from build123d import *

# Parameters (mm, degrees)
BOSS_EXTRUDE2_DEPTH     = 20
CUT_EXTRUDE1_DEPTH      = 4.016802691
CUT_EXTRUDE1_DEPTH_BACK = 7.783143762
FILLET1_R               = 3


with BuildPart() as part:
    # Sketch2 → Boss-Extrude2 (new body)
    with BuildSketch(Plane(origin=(0, 0, 0), x_dir=(1, 0, 0), z_dir=(0, 1, 0))):
        Polygon((0, 0), (-64, 6.783143762), (-64, 3.766341072), (0, -3.016802691), (64.316188922, 3.799852867), (64, 6.783143762), align=None)
    extrude(amount=BOSS_EXTRUDE2_DEPTH)

    # Sketch3 → Cut-Extrude1 (cut, two sides)
    with BuildSketch(Plane.XY) as cut_extrude1_sk:
        Polygon((0, 7.890942367), (-64, 5.798881402), (-64, 0), (64.316188922, 0), (64.316188922, 5.838536205), align=None)
        Polygon((-64, 20), (-64, 15.798881402), (0, 17.890942367), (64.316188922, 15.838536205), (64.316188922, 20), align=None)
    extrude(amount=CUT_EXTRUDE1_DEPTH, mode=Mode.SUBTRACT)
    extrude(cut_extrude1_sk.sketch, amount=-CUT_EXTRUDE1_DEPTH_BACK, mode=Mode.SUBTRACT)

    # Fillet1
    fillet1_edges = [part.edges().sort_by_distance(p)[0] for p in [
        (64.158094461, 15.843581188, -5.291498315),
        (64.158094461, 5.843581188, -5.291498315),
        (-64, 5.798881402, -5.274742417),
        (-64, 15.798881402, -5.274742417),
    ]]
    fillet(fillet1_edges, radius=FILLET1_R)


solid = part.part
Can you work these out from the model? Positions are in its coordinate system, mm. A direction names the side the tool comes from. Coordinates: 2 decimals unless noted, no trailing zeros. Write each loop counter-clockwise with the first axis right and the second up, starting at its lowest first coordinate (ties: lowest second). Pieces come first, ordered by that corner, then holes. Notation, with made-up numbers: (-6.75, 36.5) -> (32.25, 36.5) arc R21 cw to (32.25, 41.5) -> close; hole circle Ø11 at (44.25, 35). An arc over 180 degrees is marked (long way). Write each question's results on one line, items separated by ' | '. Start each with the question number.
Q1. Imagine slicing it at B-B (z = 1.75). Write out the boundary of the cut face in (x, y).
Q2. Imagine slicing it at C-C (x = -48.5). Write out the boundary of the cut face in (y, z).
Q3. Imagine slicing it at A-A (y = 10.75). Write out the boundary of the cut face in (x, z), then the cut area to 3 significant figures.
Q4. On a 3-axis mill with a long thin cutter (end or side, diameter ignored), from which of +Z, -Z, +X, -X, +Y, -Y can I reach the whole of each face in a straight line? I mean faces 4 (the face through (32.45, 11.83, -3.44)), 5 (the face through (31.708, 11.829, -0.344)). Say none if no direction works.
Q5. If I drill on probe 1 along Z at (x, y) = (-14.5, 14); probe 2 along Z at (x, y) = (-19, 11.75); probe 3 along Y at (x, z) = (-8, 1.5), over which ranges is the centre line in solid material (lowest first)?
Q6. We'd pull the mould along X, two halves only. Please class faces 1 (the face through (-31.552, 11.811, -3.344)), 2 (the face through (-64, 11, -5)), 3 (the face through (64.16, 10.91, -5.27)): +X half, -X half, draft (parallel to the pull), parting line (faces both ways), or undercut.
Q7. I'm going to push flat-ended pins straight in: pin 1 (2 mm diameter, centred on x = 30, z = 0.5, fed in from +Y); pin 2 (4 mm diameter, centred on x = 25, y = 13.5, fed in from +Z); pin 3 (1 mm diameter, centred on x = -47, y = 9, fed in from +Z). Where does each tip first touch, or does it pass through?
Taken from the geometry:
1) outline: (-11.95, 7.5) -> (0, 7.89) -> (11.95, 7.51) -> (11.95, 17.51) -> (0, 17.89) -> (-11.95, 17.5) -> close
2) outline: (6.31, -5.14) -> (16.31, -5.14) -> (16.31, -2.12) -> (6.31, -2.12) -> close
3) outline: (-64, -6.78) -> (0, 0) -> (64, -6.78) -> (64.32, -3.8) -> (0, 3.02) -> (-64, -3.77) -> close | area: 387 mm^2
4) face 4: -Z, +Y, -Y | face 5: +Z, +X, +Y, -Y
5) probe 1: z = -1.54 to 1.48 | probe 2: z = -2.01 to 1 | probe 3: y = 7.63 to 17.63
6) face 1: undercut | face 2: -X half | face 3: +X half
7) pin 1: stops at y = 16.96 | pin 2: stops at z = 0.58 | pin 3: stops at z = -1.91
